```python
from build123d import *

# Parameters (mm, degrees)
SKETCH1_W                = 203.2
SKETCH1_H                = 304.8
BOSS_EXTRUDE1_DEPTH      = 19.05
ESQUISSE2_W              = 203.2
ESQUISSE2_H              = 38.1
ENL_V_MAT_EXTRU_2_DEPTH  = 367.819005097
ESQUISSE3_W              = 203.2
ESQUISSE3_H              = 93.472
ENL_V_MAT_EXTRU_3_DEPTH  = 336.830362683
ESQUISSE5_R              = 19.2405
ENL_V_MAT_EXTRU_5_DEPTH  = 268.695876853
ESQUISSE9_R              = 10.9982
ENL_V_MAT_EXTRU_9_DEPTH  = 6.985
ESQUISSE10_R             = 6.35
ENL_V_MAT_EXTRU_10_DEPTH = 268.289626078
ESQUISSE11_W             = 60.452
ESQUISSE11_H             = 12.7
ENL_V_MAT_EXTRU_11_DEPTH = 19.05


with BuildPart() as part:
    # Sketch1 → Boss-Extrude1 (new body)
    with BuildSketch(Plane.XY):
        with Locations((101.6, 152.4)):
            Rectangle(SKETCH1_W, SKETCH1_H)
    extrude(amount=BOSS_EXTRUDE1_DEPTH)

    # Esquisse2 → Enlèv. mat.-Extru.2 (cut, through all)
    with BuildSketch(Plane(origin=(0, 0, 0), x_dir=(-1, 0, 0), z_dir=(0, 0, -1))):
        with Locations((-101.6, 285.75)):
            Rectangle(ESQUISSE2_W, ESQUISSE2_H)
    extrude(amount=-ENL_V_MAT_EXTRU_2_DEPTH, mode=Mode.SUBTRACT)

    # Esquisse3 → Enlèv. mat.-Extru.3 (cut, through all)
    with BuildSketch(Plane(origin=(0, 0, 0), x_dir=(-1, 0, 0), z_dir=(0, 0, -1))):
        with Locations((-101.6, 219.964)):
            Rectangle(ESQUISSE3_W, ESQUISSE3_H)
    extrude(amount=-ENL_V_MAT_EXTRU_3_DEPTH, mode=Mode.SUBTRACT)

    # Esquisse5 → Enlèv. mat.-Extru.5 (cut, through all)
    with BuildSketch(Plane(origin=(0, 0, 0), x_dir=(-1, 0, 0), z_dir=(0, 0, -1))):
        with Locations((-174.498, 144.526)):
            Circle(ESQUISSE5_R)
        with Locations((-28.702, 144.526)):
            Circle(ESQUISSE5_R)
    extrude(amount=-ENL_V_MAT_EXTRU_5_DEPTH, mode=Mode.SUBTRACT)

    # Esquisse9 → Enlèv. mat.-Extru.9 (cut)
    with BuildSketch(Plane.XY.offset(19.05)):
        with Locations((101.6, 144.526)):
            Circle(ESQUISSE9_R)
    extrude(amount=-ENL_V_MAT_EXTRU_9_DEPTH, mode=Mode.SUBTRACT)

    # Esquisse10 → Enlèv. mat.-Extru.10 (cut, through all)
    with BuildSketch(Plane.XY.offset(12.065)):
        with Locations((101.6, 144.526)):
            Circle(ESQUISSE10_R)
    extrude(amount=-ENL_V_MAT_EXTRU_10_DEPTH, mode=Mode.SUBTRACT)

    # Esquisse11 → Enlèv. mat.-Extru.11 (cut)
    with BuildSketch(Plane(origin=(0, 0, 0), x_dir=(-1, 0, 0), z_dir=(0, 0, -1))):
        with Locations((-101.6, 166.878)):
            Rectangle(ESQUISSE11_W, ESQUISSE11_H)
    extrude(amount=-ENL_V_MAT_EXTRU_11_DEPTH, mode=Mode.SUBTRACT)


solid = part.part
```
Geometry: final body of the model. Coordinates: model frame, mm. A direction names the side the tool comes from. Round coordinates to 2 decimals unless told otherwise and drop trailing zeros. Loops run counter-clockwise (first coordinate to the right, second up) from the corner with the lowest first, then second, coordinate; pieces in that order, holes last. Notation, with made-up numbers: (56, -22.5) -> (107, -22.5) arc R12 ccw to (107, -0.5) -> close; hole circle Ø1 at (-24, -18). An arc over 180 degrees is marked (long way). Write each question's results on one line, items separated by ' | '.
Item 1: Pin query (flat end, axial travel): pin 1 Ø10 at (x, y) = (101.6, 144.526) entering from +Z; pin 2 Ø9.5 at (x, z) = (114, 10) entering from +Y; pin 3 Ø6.5 at (x, y) = (104, 142) entering from +Z (3 decimals). Return the tip coordinate at first contact, or that it passes through.
Answers below:
pin 1: passes through | pin 2: stops at y = 160.53 | pin 3: stops at z = 12.065
Item 2: Cut plane D-D on x = 187. Return the cut outline in (y, z).
Answers below:
outline: (0, 0) -> (129.9, 0) -> (129.9, 19.05) -> (0, 19.05) -> close; (159.15, 0) -> (173.23, 0) -> (173.23, 19.05) -> (159.15, 19.05) -> close
Item 3: Cut plane B-B on y = 158. Return the cut outline in (x, z), and give its area (3 significant figures).
Answers below:
outline: (0, 0) -> (14.97, 0) -> (14.97, 19.05) -> (0, 19.05) -> close; (42.44, 0) -> (160.76, 0) -> (160.76, 19.05) -> (42.44, 19.05) -> close; (188.23, 0) -> (203.2, 0) -> (203.2, 19.05) -> (188.23, 19.05) -> close | area: 2,820 mm²
Item 4: Set-up query: faces 5 (the face through (131.826, 167, 9)), 6 (the face through (99.22, 133.79, 15.61)), 7 (the face through (107.657, 146.433, 6.117)). Return all of +Z, -Z, +X, -X, +Y, -Y with unobstructed straight access to the full face (end or side cutting, diameter ignored); none if empty.
Answers below:
face 5: +Z, -Z, +Y | face 6: +Z | face 7: +Z, -Z
Item 5: Cut plane A-A on x = 101.6. Return the cut outline in (y, z) (3 decimals).
Answers below:
outline: (0, 0) -> (138.176, 0) -> (138.176, 12.065) -> (133.528, 12.065) -> (133.528, 19.05) -> (0, 19.05) -> close; (150.876, 0) -> (160.528, 0) -> (160.528, 19.05) -> (155.524, 19.05) -> (155.524, 12.065) -> (150.876, 12.065) -> close
Item 6: Line query: probe 1 along Y at (x, z) = (101.6, 14); probe 2 along Y at (x, z) = (173.5, 16); probe 3 along Y at (x, z) = (124, 9.25). Output: solid intervals per line, ascending. Write a range as [from, to].
Answers below:
probe 1: y = [0, 133.53], [155.52, 160.53] | probe 2: y = [0, 125.31], [163.74, 173.23] | probe 3: y = [0, 160.53]
Item 7: Cut plane C-C on z = 3.5. Return the cut outline in (x, y), and give its area (3 significant figures).
Answers below:
outline: (0, 0) -> (203.2, 0) -> (203.2, 173.23) -> (131.83, 173.23) -> (131.83, 160.53) -> (71.37, 160.53) -> (71.37, 173.23) -> (0, 173.23) -> close; hole circle Ø38.48 at (28.7, 144.53); hole circle Ø12.7 at (101.6, 144.53); hole circle Ø38.48 at (174.5, 144.53) | area: 32,000 mm²
Item 8: Pull-direction query (X, two-part tool) for faces 1 (the face through (0, 85, 9)), 2 (the face through (102, 160.528, 9)), 3 (the face through (100, 0, 9)), 4 (the face through (203.2, 85, 9)); classes: pulls with the +X half, pulls with the -X half, needs draft (parallel to the pull), parting line crosses it, or undercut.
Answers below:
face 1: pulls with the -X half | face 2: undercut | face 3: needs draft | face 4: pulls with the +X half
